Model file for the job. Use its own axes, mm. Face numbers are marked on the shaded views. A direction names the side the tool comes from. Give positions to 0.01 mm unless a question says otherwise; leave off trailing zeros. Order: outer loops, then holes, each group sorted by start corner. A loop starts at its lowest first (then second) coordinate and runs counter-clockwise, first axis right, second up. Notation, with made-up numbers: M -11.5,-37 L 29.5,-37 A19 ccw 29.5,-28 Z; hole C 35.25,4.25 d8. An arc over 180 degrees is marked long. Return JSON: item names as keys, results as strings. Group by question number.
1. Slice it at C-C on x = -5.5. List the corners of the cut face in (y, z).
2. 3-axis set-ups, long thin cutter, end or side, ignore diameter. For the marked faces 1 and 2: which of +Z, -Z, +X, -X, +Y, -Y reach the whole face in a straight line?
3. Slice it at B-B on y = 194.5. List the corners of the cut face in (x, z), then the cut area to 3 significant figures.
4. Wall check: probe 1 along Z at (x, y) = (-10, 314); probe 2 along X at (y, z) = (346, 13.5). Give the ranges that are in metal, low to high. Write a range as [from, to].
5. Slice it at A-A on z = 12. List the corners of the cut face in (x, y), then the cut area to 3 significant figures.
6. Two-plate mould, pull along X, no slides. Class the marked faces 3, 4 and 5: released by +X, released by -X, zero draft, split by the parting line, or undercut.
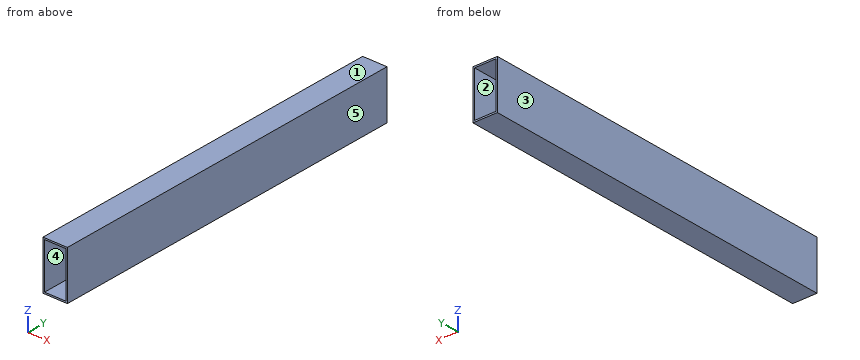
from build123d import *

# Parameters (mm, degrees)
SKETCH1_W               = 25.4
SKETCH1_H               = 50.8
BOSS_EXTRUDE1_DEPTH     = 384.556
CUT_EXTRUDE1_DEPTH      = 386.603121274
CUT_EXTRUDE1_DEPTH_BACK = 386.603121274
SKETCH2_W               = 22.098
SKETCH2_H               = 47.498


with BuildPart() as part:
    # Sketch1 → Boss-Extrude1 (new body)
    with BuildSketch(Plane(origin=(0, 0, 0), x_dir=(1, 0, 0), z_dir=(0, 1, 0))):
        Rectangle(SKETCH1_W, SKETCH1_H)
    extrude(amount=BOSS_EXTRUDE1_DEPTH)

    # Sketch2 → Cut-Extrude1 (cut, two sides: drawn at the far end of the back side and taken through both)
    with BuildSketch(Plane.XZ.offset(-CUT_EXTRUDE1_DEPTH_BACK)):
        Rectangle(SKETCH2_W, SKETCH2_H)
    extrude(amount=CUT_EXTRUDE1_DEPTH + CUT_EXTRUDE1_DEPTH_BACK, mode=Mode.SUBTRACT)


solid = part.part
Result:
{
 "1": {"outline": "M 0,-25.4 L 384.56,-25.4 L 384.56,-23.75 L 0,-23.75 Z; M 0,23.75 L 384.56,23.75 L 384.56,25.4 L 0,25.4 Z"},
 "2": {"face 1": "+Z, +X, -X, +Y, -Y", "face 2": "+Y, -Y"},
 "3": {"outline": "M -12.7,-25.4 L 12.7,-25.4 L 12.7,25.4 L -12.7,25.4 Z; hole M -11.05,-23.75 L 11.05,-23.75 L 11.05,23.75 L -11.05,23.75 Z", "area": "241 mm2"},
 "4": {"probe 1": "z = [-25.4, -23.75], [23.75, 25.4]", "probe 2": "x = [-12.7, -11.05], [11.05, 12.7]"},
 "5": {"outline": "M -12.7,0 L -11.05,0 L -11.05,384.56 L -12.7,384.56 Z; M 11.05,0 L 12.7,0 L 12.7,384.56 L 11.05,384.56 Z", "area": "1,270 mm2"},
 "6": {"face 3": "released by -X", "face 4": "undercut", "face 5": "released by +X"}
}
